The figure shows three views and two pictorial views of one solid part (mm, origin at its lowest corner). Answer the questions. Coordinates: 2 decimals unless noted, no trailing zeros. Write each loop counter-clockwise with the first axis right and the second up, starting at its lowest first coordinate (ties: lowest second). Pieces come first, ordered by that corner, then holes.
Item 1: Each of these flat-tipped pins is pushed along its axis until it touches: P1, Ø3, axis at x = 53.5, y = 76, coming from the -Z side; P2, Ø4, axis at x = 126.04, y = 25.09, coming from the -Z side; P3, Ø1, axis at y = 16, z = 2, coming from the -X side (1 decimal). Where does it stop, or does it pass through?
Item 2: Straight lines are drawn through the part: probe 1 along X at (y, z) = (98, 1.4); probe 2 along Y at (x, z) = (13.5, 4.45); probe 3 along Y at (x, z) = (32, 4.1). For each, find the intervals that lie inside material, in ascending order.
Item 3: Section B-B (x = 62) is taken. Give the vertices of the cut face in (y, z).
Item 4: Section A-A (z = 2.15) is taken. State how many separate pieces and enclosed holes the cut face has, then the cut area to 3 significant figures.
Item 5: Section C-C (y = 59.5) is taken. Give the vertices of the cut face in (x, z), then the cut area to 3 significant figures.
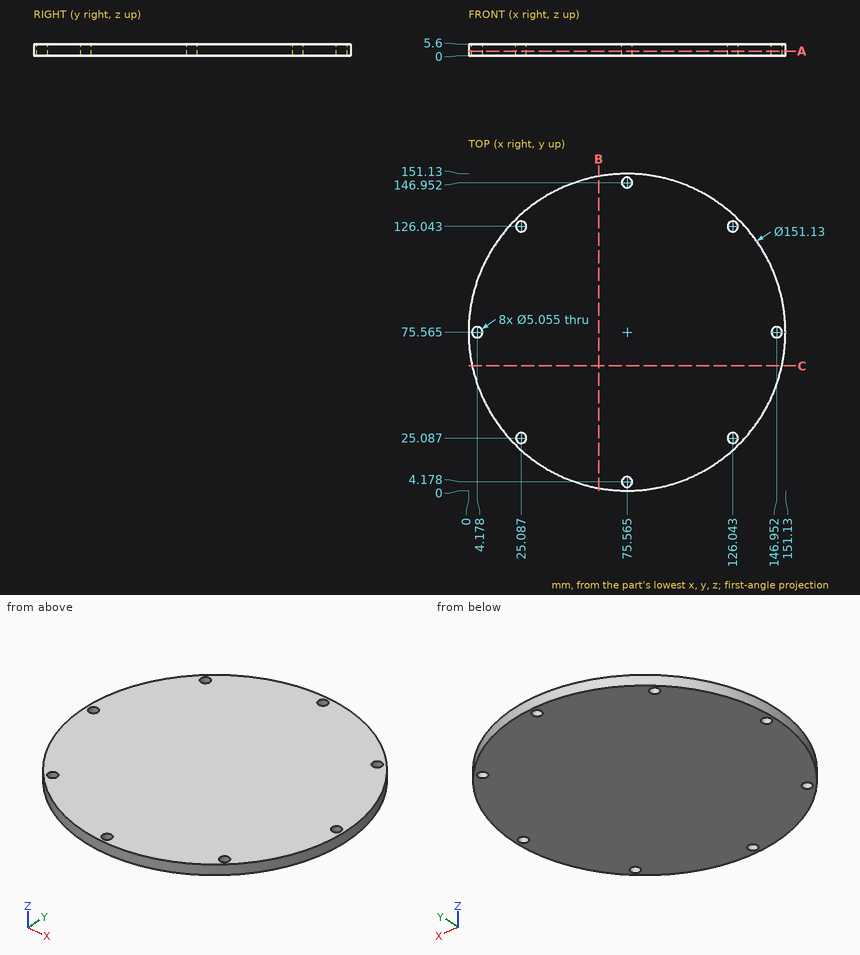
Established:
1. P1: stops at z = 0
1. P2: passes through
1. P3: stops at x = 28.4
2. probe 1: x = 3.41 to 147.72
2. probe 2: y = 32.46 to 118.67
2. probe 3: y = 13.82 to 137.31
3. outline: (1.23, 0) - (149.9, 0) - (149.9, 5.6) - (1.23, 5.6) - close
4. separate pieces: 1
4. enclosed holes: 8
4. area: 17,800 mm2
5. outline: (1.73, 0) - (149.4, 0) - (149.4, 5.6) - (1.73, 5.6) - close
5. area: 827 mm2
